The listing builds one solid part. Answer for the finished solid, in the listing's coordinates (mm). A direction names the side the tool comes from. Give positions to 0.01 mm unless a question says otherwise; leave off trailing zeros. Order: outer loops, then holes, each group sorted by start corner. A loop starts at its lowest first (then second) coordinate and runs counter-clockwise, first axis right, second up. Notation, with made-up numbers: (89.5, 47) - (115.5, 47) arc R19 cw to (115.5, 56) - close; hole circle Ø5 at (53.25, 1). An arc over 180 degrees is marked (long way). Answer in a Markdown table with one row per item.
from build123d import *

# Parameters (mm, degrees)
SKETCH2_W            = 29
SKETCH2_H            = 15.11
BOSS_EXTRUDE1_DEPTH  = 2
SKETCH7_W            = 45
SKETCH7_H            = 2
BOSS_EXTRUDE2_DEPTH  = 15
M2_CLEARANCE_HOLE1_D = 2.4
M2_CLEARANCE_HOLE2_D = 2.4


with BuildPart() as part:
    # Sketch2 → Boss-Extrude1 (new body)
    with BuildSketch(Plane(origin=(0, 0, 0), x_dir=(1, 0, 0), z_dir=(0, 1, 0))):
        with Locations((-24.397211382, -7.555)):
            Rectangle(SKETCH2_W, SKETCH2_H)
    extrude(amount=BOSS_EXTRUDE1_DEPTH)

    # Sketch7 → Boss-Extrude2 (add)
    with BuildSketch(Plane(origin=(0, 0, 0), x_dir=(-1, 0, 0), z_dir=(0, -1, 0))):
        with Locations((24.397211382, 0.886680676)):
            Rectangle(SKETCH7_W, SKETCH7_H)
    extrude(amount=-BOSS_EXTRUDE2_DEPTH)

    # M2 Clearance Hole1 (through all)
    with Locations(Plane.XY.offset(0.113319324)):
        with Locations((-42.897211382, 4)):
            Hole(M2_CLEARANCE_HOLE1_D / 2)

    # M2 Clearance Hole2 (through all)
    with Locations(Plane.XY.offset(0.113319324)):
        with Locations((-5.897211382, 4)):
            Hole(M2_CLEARANCE_HOLE2_D / 2)


solid = part.part
Item 1: Determine the mould class of faces 4 (the face through (-25, 1, 15.11)), 5 (the face through (-44.006, 3.54, -0.901)), 6 (the face through (-38.897, 1, 8)), 7 (the face through (-7.04, 4.36, -0.9)) for opening direction X: pulls with the +X half, pulls with the -X half, needs draft (parallel to the pull), parting line crosses it, or undercut.
Answer block:
| item | result |
|---|---|
| face 4 | needs draft |
| face 5 | undercut |
| face 6 | pulls with the -X half |
| face 7 | undercut |
Item 2: Which of the six approach directions +Z, -Z, +X, -X, +Y, -Y give full straight-line access (tool end or side, diameter ignored) to faces 1 (the face through (-9.897, 1, 8)), 2 (the face through (-25, 2, 8)), 3 (the face through (-1.897, 7, -1))?
Answer block:
| item | result |
|---|---|
| face 1 | +Z, +X, +Y, -Y |
| face 2 | +Z, +X, -X, +Y |
| face 3 | +Z, -Z, +X, +Y, -Y |
Item 3: Find section B-B on x = -6.5. Write down the section's boundary in (y, z).
Answer block:
| item | result |
|---|---|
| outline | (0, -1.89) - (2.96, -1.89) - (2.96, 0.11) - (0, 0.11) - close; (5.04, -1.89) - (15, -1.89) - (15, 0.11) - (5.04, 0.11) - close |
Item 4: Find section D-D on y = 13.25. Write down the section's boundary in (x, z).
Answer block:
| item | result |
|---|---|
| outline | (-46.9, -1.89) - (-1.9, -1.89) - (-1.9, 0.11) - (-46.9, 0.11) - close |
Item 5: Find section A-A on y = 4. Write down the section's boundary in (x, z), then the cut area to 3 significant figures.
Answer block:
| item | result |
|---|---|
| outline | (-46.9, -1.89) - (-44.1, -1.89) - (-44.1, 0.11) - (-46.9, 0.11) - close; (-41.7, -1.89) - (-7.1, -1.89) - (-7.1, 0.11) - (-41.7, 0.11) - close; (-4.7, -1.89) - (-1.9, -1.89) - (-1.9, 0.11) - (-4.7, 0.11) - close |
| area | 80.4 mm² |
Item 6: Each of these flat-tipped pins is pushed along its axis until it touches: P1, Ø2, axis at x = -22, y = 3.5, coming from the +Z side; P2, Ø2, axis at x = -15.5, z = 6.5, coming from the +Y side; P3, Ø1.4, axis at x = -5.9, y = 4, coming from the -Z side; P4, Ø1.6, axis at y = 1, z = 4, coming from the +X side. Where does it stop, or does it pass through?
Answer block:
| item | result |
|---|---|
| P1 | z = 0.11 |
| P2 | y = 2 |
| P3 | through |
| P4 | x = -9.9 |
Item 7: Find section C-C on x = -36. Write down the section's boundary in (y, z), then the cut area to 3 significant figures.
Answer block:
| item | result |
|---|---|
| outline | (0, -1.89) - (15, -1.89) - (15, 0.11) - (2, 0.11) - (2, 15.11) - (0, 15.11) - close |
| area | 60.0 mm² |
Item 8: Consider line 1 (Z direction, x = -14, y = 6.25); line 2 (Y direction, x = -23.5, z = 8.5). Determine where each line is inside the solid, lowest interval first.
Answer block:
| item | result |
|---|---|
| line 1 | -1.89 to 0.11 |
| line 2 | 0 to 2 |
